Input: part model. Units: mm. Frame: model coordinates. A direction names the side the tool comes from. Round coordinates to 2 decimals unless told otherwise and drop trailing zeros. Write each loop counter-clockwise with the first axis right and the second up, starting at its lowest first coordinate (ties: lowest second). Pieces come first, ordered by that corner, then holes. Notation, with made-up numbers: M 6,8.25 L 23,8.25 A14 cw 23,27.25 Z; hole C 28,74 d10. An arc over 180 degrees is marked long. Write each question's results on one line, items separated by ' | '. Start each with the question number.
```python
from build123d import *

# Parameters (mm, degrees)
F0_R     = 11.025
F1_DEPTH = 7


with BuildPart() as f1:
    # F0 (on Top) → F1 (new body)
    with BuildSketch(Plane.XY):
        with BuildLine():
            Line((8.4852813742, 26.7863036134), (0, 35.2715849876))
            Line((0, 35.2715849876), (-8.4852813742, 26.7863036134))
            Line((-8.4852813742, 26.7863036134), (-2.4852813742, 26.7863036134))
            Line((-2.4852813742, 26.7863036134), (-2.4852813742, 16.7863036134))
            ThreePointArc((-2.4852813742, 16.7863036134), (-11.2157675105, 11.2157675105), (-16.7863036134, 2.4852813742))
            Line((-16.7863036134, 2.4852813742), (-26.7863036134, 2.4852813742))
            Line((-26.7863036134, 2.4852813742), (-26.7863036134, 8.4852813742))
            Line((-26.7863036134, 8.4852813742), (-35.2715849876, 0))
            Line((-35.2715849876, 0), (-26.7863036134, -8.4852813742))
            Line((-26.7863036134, -8.4852813742), (-26.7863036134, -2.4852813742))
            Line((-26.7863036134, -2.4852813742), (-16.7863036134, -2.4852813742))
            ThreePointArc((-16.7863036134, -2.4852813742), (-11.2357756094, -11.2810159865), (-2.4852813742, -16.9025957584))
            Line((-2.4852813742, -16.9025957584), (-2.4852813742, -26.9025957584))
            Line((-2.4852813742, -26.9025957584), (-8.4852813742, -26.9025957584))
            Line((-8.4852813742, -26.9025957584), (0, -35.3878771327))
            Line((0, -35.3878771327), (8.4852813742, -26.9025957584))
            Line((8.4852813742, -26.9025957584), (2.4852813742, -26.9025957584))
            Line((2.4852813742, -26.9025957584), (2.4852813742, -16.9025957584))
            ThreePointArc((2.4852813742, -16.9025957584), (11.2357756094, -11.2810159865), (16.7863036134, -2.4852813742))
            Line((16.7863036134, -2.4852813742), (26.7863036134, -2.4852813742))
            Line((26.7863036134, -2.4852813742), (26.7863036134, -8.4852813742))
            Line((26.7863036134, -8.4852813742), (35.2715849876, 0))
            Line((35.2715849876, 0), (26.7863036134, 8.4852813742))
            Line((26.7863036134, 8.4852813742), (26.7863036134, 2.4852813742))
            Line((26.7863036134, 2.4852813742), (16.7863036134, 2.4852813742))
            ThreePointArc((16.7863036134, 2.4852813742), (11.2157675105, 11.2157675105), (2.4852813742, 16.7863036134))
            Line((2.4852813742, 16.7863036134), (2.4852813742, 26.7863036134))
            Line((2.4852813742, 26.7863036134), (8.4852813742, 26.7863036134))
        make_face()
        with BuildLine():
            Line((0.4957766307, -30.7123869197), (0.2719380573, -30.7123869197))
            Line((0.2719380573, -30.7123869197), (0.2719380573, -31.1581870135))
            Line((0.2719380573, -31.1581870135), (0.1473486626, -31.1581870135))
            Line((0.1473486626, -31.1581870135), (0.1473486626, -30.0861551036))
            Line((0.1473486626, -30.0861551036), (0.4413420929, -30.0861551036))
            add(Edge.make_bspline(
                [(0.4413420929, -30.0861551036), (0.6386672924, -30.0861551036), (0.7328718911, -30.161706488)],
                knots=[0, 0, 0, 1, 1, 1], degree=2))
            add(Edge.make_bspline(
                [(0.7328718911, -30.161706488), (0.8270764899, -30.2372578723), (0.8270764899, -30.3890645358)],
                knots=[0, 0, 0, 1, 1, 1], degree=2))
            add(Edge.make_bspline(
                [(0.8270764899, -30.3890645358), (0.8270764899, -30.6016407911), (0.6114500235, -30.6764882805)],
                knots=[0, 0, 0, 1, 1, 1], degree=2))
            Line((0.6114500235, -30.6764882805), (0.9026278742, -31.1581870135))
            Line((0.9026278742, -31.1581870135), (0.7552792116, -31.1581870135))
            Line((0.7552792116, -31.1581870135), (0.4957766307, -30.7123869197))
        make_face(mode=Mode.SUBTRACT)
        with BuildLine():
            Line((-30.4200164008, 0.0797443089), (-30.6438549742, 0.0797443089))
            Line((-30.6438549742, 0.0797443089), (-30.6438549742, -0.366055785))
            Line((-30.6438549742, -0.366055785), (-30.7684443689, -0.366055785))
            Line((-30.7684443689, -0.366055785), (-30.7684443689, 0.7059761249))
            Line((-30.7684443689, 0.7059761249), (-30.4744509385, 0.7059761249))
            add(Edge.make_bspline(
                [(-30.4744509385, 0.7059761249), (-30.2771257391, 0.7059761249), (-30.1829211403, 0.6304247406)],
                knots=[0, 0, 0, 1, 1, 1], degree=2))
            add(Edge.make_bspline(
                [(-30.1829211403, 0.6304247406), (-30.0887165415, 0.5548733563), (-30.0887165415, 0.4030666927)],
                knots=[0, 0, 0, 1, 1, 1], degree=2))
            add(Edge.make_bspline(
                [(-30.0887165415, 0.4030666927), (-30.0887165415, 0.1904904375), (-30.304343008, 0.115642948)],
                knots=[0, 0, 0, 1, 1, 1], degree=2))
            Line((-30.304343008, 0.115642948), (-30.0131651572, -0.366055785))
            Line((-30.0131651572, -0.366055785), (-30.1605138198, -0.366055785))
            Line((-30.1605138198, -0.366055785), (-30.4200164008, 0.0797443089))
        make_face(mode=Mode.SUBTRACT)
        Circle(F0_R, mode=Mode.SUBTRACT)
        with BuildLine():
            Line((31.1531984282, 0.0540223872), (30.9293598548, 0.0540223872))
            Line((30.9293598548, 0.0540223872), (30.9293598548, -0.3917777067))
            Line((30.9293598548, -0.3917777067), (30.8047704601, -0.3917777067))
            Line((30.8047704601, -0.3917777067), (30.8047704601, 0.6802542032))
            Line((30.8047704601, 0.6802542032), (31.0987638904, 0.6802542032))
            add(Edge.make_bspline(
                [(31.0987638904, 0.6802542032), (31.2960890899, 0.6802542032), (31.3902936886, 0.6047028189)],
                knots=[0, 0, 0, 1, 1, 1], degree=2))
            add(Edge.make_bspline(
                [(31.3902936886, 0.6047028189), (31.4844982874, 0.5291514346), (31.4844982874, 0.377344771)],
                knots=[0, 0, 0, 1, 1, 1], degree=2))
            add(Edge.make_bspline(
                [(31.4844982874, 0.377344771), (31.4844982874, 0.1647685158), (31.268871821, 0.0899210263)],
                knots=[0, 0, 0, 1, 1, 1], degree=2))
            Line((31.268871821, 0.0899210263), (31.5600496718, -0.3917777067))
            Line((31.5600496718, -0.3917777067), (31.4127010092, -0.3917777067))
            Line((31.4127010092, -0.3917777067), (31.1531984282, 0.0540223872))
        make_face(mode=Mode.SUBTRACT)
        with BuildLine():
            Line((0.1811846398, 30.4459987263), (-0.0426539337, 30.4459987263))
            Line((-0.0426539337, 30.4459987263), (-0.0426539337, 30.0001986325))
            Line((-0.0426539337, 30.0001986325), (-0.1672433283, 30.0001986325))
            Line((-0.1672433283, 30.0001986325), (-0.1672433283, 31.0722305424))
            Line((-0.1672433283, 31.0722305424), (0.126750102, 31.0722305424))
            add(Edge.make_bspline(
                [(0.126750102, 31.0722305424), (0.3240753015, 31.0722305424), (0.4182799002, 30.9966791581)],
                knots=[0, 0, 0, 1, 1, 1], degree=2))
            add(Edge.make_bspline(
                [(0.4182799002, 30.9966791581), (0.512484499, 30.9211277737), (0.512484499, 30.7693211102)],
                knots=[0, 0, 0, 1, 1, 1], degree=2))
            add(Edge.make_bspline(
                [(0.512484499, 30.7693211102), (0.512484499, 30.5567448549), (0.2968580326, 30.4818973655)],
                knots=[0, 0, 0, 1, 1, 1], degree=2))
            Line((0.2968580326, 30.4818973655), (0.5880358833, 30.0001986325))
            Line((0.5880358833, 30.0001986325), (0.4406872207, 30.0001986325))
            Line((0.4406872207, 30.0001986325), (0.1811846398, 30.4459987263))
        make_face(mode=Mode.SUBTRACT)
    extrude(amount=F1_DEPTH)


solid = f1.part
```
1. Access query for faces 1 (the face through (-2.485, -22, 3)), 2 (the face through (2.485, -22, 3)), 3 (the face through (-22, 2.485, 3)). Directions: +Z, -Z, +X, -X, +Y, -Y. A direction counts if a zero-diameter tool reaches every point of the face in a straight line with its end or side. Return the directions, or none.
2. Cut plane D-D on z = 3.25. Give the number of separate pieces and of enclosed holes in the cut face, and give its area (3 significant figures).
3. Cut plane B-B on y = -5. Output: boundary loops of the cut face in (x, z), and give its area (3 significant figures).
4. Line query: L1, parallel to Y at x = 0, z = 2.5 (3 decimals); L2, parallel to Y at x = -6, z = 1.75; L3, parallel to X at y = 6, z = 3. Output: solid intervals per line, ascending. Write a range as from..to.
5. Cut plane A-A on x = 5.5. Output: boundary loops of the cut face in (y, z).
6. Cut plane C-C on x = -9.5. Output: boundary loops of the cut face in (y, z).
7. Contact query for flat-ended pins moving along their axis: P1, Ø1.8, axis at y = 5, z = 2, coming from the +X side; P2, Ø4, axis at x = -4, z = 3.5, coming from the -Y side; P3, Ø3, axis at y = -25.5, z = 6, coming from the +X side. Output: stop coordinate, or through.
Answers follow:
1) face 1: +Z, -Z, -X | face 2: +Z, -Z, +X | face 3: +Z, -Z, +Y
2) separate pieces: 1 | enclosed holes: 5 | area: 946 mm2
3) outline: M -30.27,0 L -26.79,0 L -26.79,7 L -30.27,7 Z; M -15.72,0 L -9.83,0 L -9.83,7 L -15.72,7 Z; M 9.83,0 L 15.72,0 L 15.72,7 L 9.83,7 Z; M 26.79,0 L 30.27,0 L 30.27,7 L 26.79,7 Z | area: 131 mm2
4) L1: y = -35.388..-11.025, 11.025..30.446, 31.072..35.272 | L2: y = -29.39..-26.9, -15.28..-9.25, 9.25..15.17, 26.79..29.27 | L3: x = -29.27..-26.79, -15.17..-9.25, 9.25..15.17, 26.79..29.27
5) outline: M -29.89,0 L -26.9,0 L -26.9,7 L -29.89,7 Z; M -15.55,0 L -9.56,0 L -9.56,7 L -15.55,7 Z; M 9.56,0 L 15.44,0 L 15.44,7 L 9.56,7 Z; M 26.79,0 L 29.77,0 L 29.77,7 L 26.79,7 Z
6) outline: M -12.87,0 L -5.59,0 L -5.59,7 L -12.87,7 Z; M 5.59,0 L 12.77,0 L 12.77,7 L 5.59,7 Z
7) P1: stops at x = 31.17 | P2: stops at y = -33.39 | P3: stops at x = 8.49
